The model under review builds one solid part; all positions refer to its coordinate system, in mm. Face numbers are marked on the shaded views. A direction names the side the tool comes from. Round coordinates to 2 decimals unless told otherwise and drop trailing zeros. Write each loop counter-clockwise with the first axis right and the second up, starting at its lowest first coordinate (ties: lowest second). Pieces come first, ordered by that corner, then holes. Notation, with made-up numbers: M -22.5,-11.5 L 26.5,-11.5 A20 cw 26.5,1.5 Z; hole C 63,79.5 d6. An arc over 180 degrees is marked long. One line per item, written item: value. Start each with the question number.
1) Take a section at A-A, the plane x = 0. Write out the cut boundary in (y, z), and give its area (3 significant figures).
2) Mouldability with a two-part tool opening along Z and no side actions: class the marked faces 1, 2 and 3 as +Z half, -Z half, draft (parallel to the pull), parting line (faces both ways), or undercut.
3) Take a section at D-D, the plane y = 6.5. Write out the cut boundary in (x, z), and give its area (3 significant figures).
4) Wall thickness on probe 1 along X at (y, z) = (6, 0); probe 2 along Z at (x, y) = (-17, 6); probe 3 along Z at (x, y) = (0, 3): over which ranges is each line inside the solid? List them lowest first.
5) Take a section at B-B, the plane y = 3. Write out the cut boundary in (x, z) (3 decimals).
6) For P1, Ø10.5, axis at x = -17, z = 0, coming from the +Y side; P2, Ø6.5, axis at x = -1, z = 1.5, coming from the +Y side; P3, Ø4, axis at x = 18.5, z = -0.5, coming from the +Y side; P4, Ø2.5, axis at x = 17, z = 0, coming from the -Y side, all flat-tipped, find the tip position at first contact; note any pin that passes through.
7) Take a section at C-C, the plane z = 0. State how many separate pieces and enclosed holes the cut face has, and give its area (3 significant figures).
8) Tool access review of the marked faces 4 and 5: name each direction out of +Z, -Z, +X, -X, +Y, -Y from which nothing blocks a thin tool from reaching the whole face with its end or side.
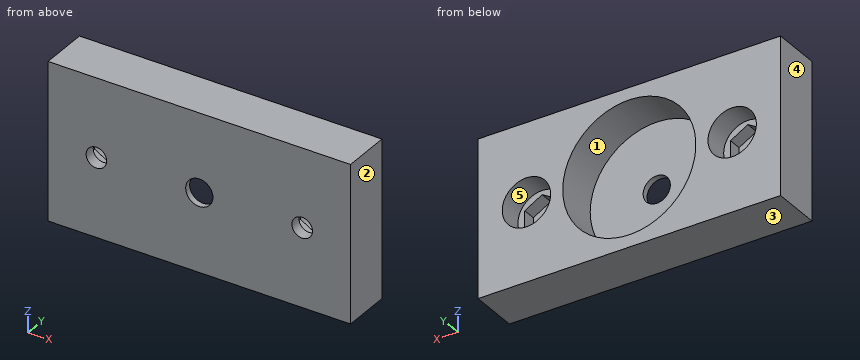
from build123d import *

# Parameters (mm, degrees)
SKETCH1_W                = 50
SKETCH1_H                = 26
BOSS_EXTRUDE1_DEPTH      = 8
SKETCH2_R                = 11
CUT_EXTRUDE1_DEPTH       = 7
SKETCH5_R                = 2.25
CUT_EXTRUDE2_DEPTH       = 2
SKETCH6_R                = 4
CUT_EXTRUDE3_DEPTH       = 4
CUT_EXTRUDE4_DEPTH       = 2.2
M3_CLEARANCE_HOLE1_D     = 3.4
M3_CLEARANCE_HOLE1_DEPTH = 1.8


with BuildPart() as part:
    # Sketch1 → Boss-Extrude1 (new body)
    with BuildSketch(Plane(origin=(0, 0, 0), x_dir=(1, 0, 0), z_dir=(0, 1, 0))):
        Rectangle(SKETCH1_W, SKETCH1_H)
    extrude(amount=BOSS_EXTRUDE1_DEPTH)

    # Sketch2 → Cut-Extrude1 (cut)
    with BuildSketch(Plane(origin=(0, 8, 0), x_dir=(1, 0, 0), z_dir=(0, 1, 0))):
        Circle(SKETCH2_R)
    extrude(amount=-CUT_EXTRUDE1_DEPTH, mode=Mode.SUBTRACT)

    # Sketch5 → Cut-Extrude2 (cut, through all)
    with BuildSketch(Plane(origin=(0, 1, 0), x_dir=(1, 0, 0), z_dir=(0, 1, 0))):
        Circle(SKETCH5_R)
    extrude(amount=-CUT_EXTRUDE2_DEPTH, mode=Mode.SUBTRACT)

    # Sketch6 → Cut-Extrude3 (cut)
    with BuildSketch(Plane(origin=(0, 8, 0), x_dir=(1, 0, 0), z_dir=(0, 1, 0))):
        with Locations((17, 0)):
            Circle(SKETCH6_R)
        with Locations((-17, 0)):
            Circle(SKETCH6_R)
    extrude(amount=-CUT_EXTRUDE3_DEPTH, mode=Mode.SUBTRACT)

    # Sketch7 → Cut-Extrude4 (cut)
    with BuildSketch(Plane(origin=(0, 4, 0), x_dir=(1, 0, 0), z_dir=(0, 1, 0))):
        Polygon((19.875, -1.659882024), (19.875, 1.659882024), (17, 3.319764048), (14.125, 1.659882024), (14.125, -1.659882024), (17, -3.319764048), align=None)
        Polygon((-17, -3.319764048), (-19.875, -1.659882024), (-19.875, 1.659882024), (-17, 3.319764048), (-14.125, 1.659882024), (-14.125, -1.659882024), align=None)
    extrude(amount=-CUT_EXTRUDE4_DEPTH, mode=Mode.SUBTRACT)

    # M3 Clearance Hole1
    with Locations(Plane(origin=(0, 1.8, 0), x_dir=(1, 0, 0), z_dir=(0, 1, 0))):
        with Locations((17, 0), (-17, 0)):
            Hole(M3_CLEARANCE_HOLE1_D / 2, depth=M3_CLEARANCE_HOLE1_DEPTH)


solid = part.part
Checked values:
1. outline: M 0,-13 L 8,-13 L 8,-11 L 1,-11 L 1,-2.25 L 0,-2.25 Z; M 0,2.25 L 1,2.25 L 1,11 L 8,11 L 8,13 L 0,13 Z
1. area: 49.5 mm2
2. face 1: undercut
2. face 2: draft
2. face 3: -Z half
3. outline: M -25,-13 L 25,-13 L 25,13 L -25,13 Z; hole C -17,0 d8; hole C 0,0 d22; hole C 17,0 d8
3. area: 819 mm2
4. probe 1: x = -25 to -21, -13 to -11, 11 to 13, 21 to 25
4. probe 2: z = -13 to -4, 4 to 13
4. probe 3: z = -13 to -11, 11 to 13
5. outline: M -25,-13 L 25,-13 L 25,13 L -25,13 Z; hole M -19.875,-1.66 L -17,-3.32 L -14.125,-1.66 L -14.125,1.66 L -17,3.32 L -19.875,1.66 Z; hole C 0,0 d22; hole M 14.125,-1.66 L 17,-3.32 L 19.875,-1.66 L 19.875,1.66 L 17,3.32 L 14.125,1.66 Z
6. P1: stops at y = 8
6. P2: stops at y = 1
6. P3: stops at y = 4
6. P4: passes through
7. separate pieces: 4
7. enclosed holes: 0
7. area: 140 mm2
8. face 4: +Z, -Z, -X, +Y, -Y
8. face 5: +Y
